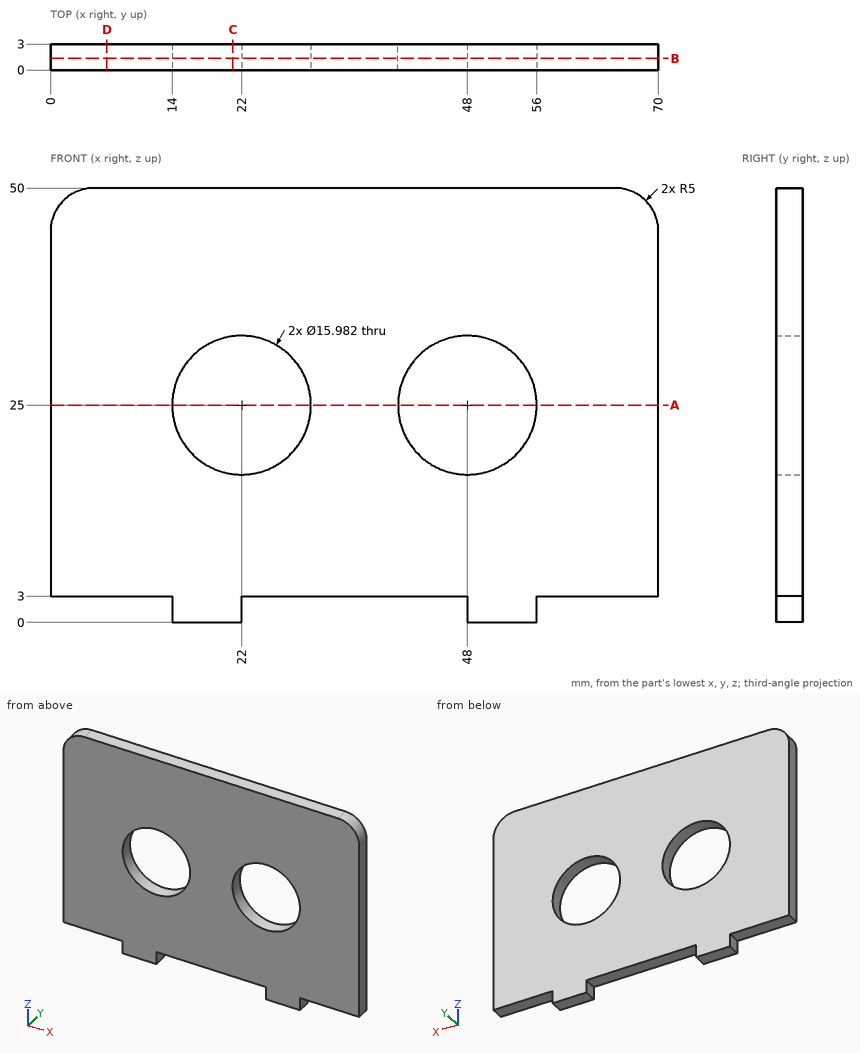
The figure shows three views and two pictorial views of one solid part (mm, origin at its lowest corner). Answer the questions. Round coordinates to 2 decimals unless told otherwise and drop trailing zeros. Write each loop counter-clockwise with the first axis right and the second up, starting at its lowest first coordinate (ties: lowest second). Pieces come first, ordered by that corner, then holes. Notation, with made-up numbers: (-18.75, 75) -> (0.25, 75) arc R14 ccw to (0.25, 100) -> close; hole circle Ø10 at (83.25, 51). An arc over 180 degrees is marked (long way). Write each question's results on one line, items separated by ' | '.
Q1. Section D-D, the plane x = 6.5 is taken. Write down the section's boundary in (y, z).
Data:
outline: (0, 3) -> (3, 3) -> (3, 50) -> (0, 50) -> close
Q2. Flat-ended cylindrical pins translate along their axes: P1, Ø1.5, axis at y = 1, z = 1, coming from the -X side; P2, Ø1.5, axis at y = 1.5, z = 2, coming from the +X side. Find the tip coordinate at first contact, or state that the pin passes through.
Data:
P1: x = 14 | P2: x = 56
Q3. Section B-B, the plane y = 1.35 is taken. Write down the section's boundary in (x, z).
Data:
outline: (0, 3) -> (14, 3) -> (14, 0) -> (22, 0) -> (22, 3) -> (48, 3) -> (48, 0) -> (56, 0) -> (56, 3) -> (70, 3) -> (70, 45) arc R5 ccw to (65, 50) -> (5, 50) arc R5 ccw to (0, 45) -> close; hole circle Ø15.98 at (22, 25); hole circle Ø15.98 at (48, 25)
Q4. Straight lines are drawn through the part: line 1 along X through (y, z) = (0.5, 19); line 2 along Z through (x, y) = (52.5, 2.1); line 3 along Z through (x, y) = (33.5, 1.7). For each, find the intervals that lie inside material, in ascending order. Write a range as [from, to].
Data:
line 1: [0, 16.72], [27.28, 42.72], [53.28, 70] | line 2: [0, 18.4], [31.6, 50] | line 3: [3, 50]
Q5. Section A-A, the plane z = 25 is taken. Write down the section's boundary in (x, y), then the cut area to 3 significant figures.
Data:
outline: (0, 0) -> (14.01, 0) -> (14.01, 3) -> (0, 3) -> close; (29.99, 0) -> (40.01, 0) -> (40.01, 3) -> (29.99, 3) -> close; (55.99, 0) -> (70, 0) -> (70, 3) -> (55.99, 3) -> close | area: 114 mm^2
Q6. Section C-C, the plane x = 21 is taken. Write down the section's boundary in (y, z), then the cut area to 3 significant figures.
Data:
outline: (0, 0) -> (3, 0) -> (3, 17.07) -> (0, 17.07) -> close; (0, 32.93) -> (3, 32.93) -> (3, 50) -> (0, 50) -> close | area: 102 mm^2
